Check sheet for the modelled part. Datum: model origin and axes. Units: mm. Round coordinates to 2 decimals unless told otherwise and drop trailing zeros. Order: outer loops, then holes, each group sorted by start corner. A loop starts at its lowest first (then second) coordinate and runs counter-clockwise, first axis right, second up.
from build123d import *

# Parameters (mm, degrees)
F1_DEPTH = 6.35
F2_DEPTH = 6.35
F3_SIZE2 = 6.34999
F3_SIZE  = 6.34999
F4_DEPTH = 0.127
F5_DEPTH = 0.127
F7_DEPTH = 0.254
F8_DEPTH = 12.954


# Not quite as in the source:
# - a fillet or chamfer is up to 0.001 mm smaller than in the source, because OpenCascade refuses the exact size


with BuildPart() as f1:
    # F0 (on Front) → F1 (new body)
    with BuildSketch(Plane.XZ):
        Polygon((-17.139416188, 28.1973872334), (-27.9807504267, 3.4191238228), (0, -37.7674587071), (27.964355424, 3.4191238228), (17.08493568, 28.1973872334), (17.08493568, 469.1244959831), (0, 506.7884922028), (-17.139416188, 469.1244959831), align=None)
    extrude(amount=F1_DEPTH)

    # F2 (add): a face of the model
    f2_faces = [f1.faces().sort_by_distance(p)[0] for p in [
        (-0.0248835797, 0, 225.9211420486),
    ]]
    extrude(f2_faces, amount=F2_DEPTH)

    # F3 (size 6.35 and 6.35 in the source; OpenCascade refuses exactly that, so slightly less here)
    f3_edges = [f1.edges().sort_by_distance(p)[0] for p in [
        (-22.560083, -6.35, 15.808256),
        (-13.990375, -6.35, -17.174167),
        (13.982178, -6.35, -17.174167),
        (22.524646, -6.35, 15.808256),
        (17.084936, -6.35, 248.660942),
        (8.542468, -6.35, 487.956494),
        (-8.569708, -6.35, 487.956494),
        (-17.139416, -6.35, 248.660942),
        (-22.560083, 6.35, 15.808256),
        (-13.990375, 6.35, -17.174167),
        (13.982178, 6.35, -17.174167),
        (22.524646, 6.35, 15.808256),
        (17.084936, 6.35, 248.660942),
        (8.542468, 6.35, 487.956494),
        (-8.569708, 6.35, 487.956494),
        (-17.139416, 6.35, 248.660942),
    ]]
    chamfer(f3_edges, length=F3_SIZE, length2=F3_SIZE2)

    # F4 (cut): a face of the model
    f4_faces = [f1.faces().sort_by_distance(p)[0] for p in [
        (-0.0252861091, -6.35, 223.0026633937),
    ]]
    extrude(f4_faces, amount=-F4_DEPTH, mode=Mode.SUBTRACT)

    # F5 (cut): a face of the model
    f5_faces = [f1.faces().sort_by_distance(p)[0] for p in [
        (-0.0252861091, 6.35, 223.0026633937),
    ]]
    extrude(f5_faces, amount=-F5_DEPTH, mode=Mode.SUBTRACT)

    # F6 (on face) → F7 (join)
    with BuildSketch(Plane.XZ.offset(6.223)):
        Polygon((8.6913099512, 0), (0, 17.8065411747), (-8.6860535666, 0), (0, -17.7944861352), align=None)
    extrude(amount=F7_DEPTH)

    # F8 (add): a face of the model
    f8_faces = [f1.faces().sort_by_distance(p)[0] for p in [
        (0.0017521282, -6.477, 0.0040183465),
    ]]
    extrude(f8_faces, amount=-F8_DEPTH)


solid = f1.part
1) Scan lines: line 1 (Y direction, x = -4, z = 74); line 2 (X direction, y = -2.5, z = 204); line 3 (Y direction, x = 15, z = 249). Record each from-to range of solid material in increasing order.
2) Gauge pin test, flat ends, axial feed: pin 1 (1.5 mm diameter, centred on x = 2, z = 246.5, fed in from +Y); pin 2 (5 mm diameter, centred on x = 2.5, y = 1, fed in from -Z); pin 3 (2 mm diameter, centred on y = -4.5, z = 208, fed in from +X). Record the tip position at first contact, or that the pin passes through.
3) Sectioned sample at B-B on y = 2.5. Record the cut outline in (x, z), and give its area (3 significant figures).
Values found:
1. line 1: y = -6.22 to 6.22
1. line 2: x = -14.64 to 14.58
1. line 3: y = -2.08 to 2.08
2. pin 1: stops at y = 6.22
2. pin 2: stops at z = -37.46
2. pin 3: stops at x = 13.58
3. outline: (-25.14, 3.68) - (0, -33.32) - (25.12, 3.68) - (14.58, 27.67) - (14.58, 468.58) - (0, 500.74) - (-14.64, 468.58) - (-14.64, 27.67) - close
3. area: 15,200 mm2
